```python
from build123d import *

# Parameters (mm, degrees)
SKETCH1_R           = 19
BOSS_EXTRUDE1_DEPTH = 32.5
CUT_EXTRUDE3_REACH  = 63.5
SKETCH2_R           = 5
CUT_EXTRUDE4_DEPTH  = 4.5


with BuildPart() as part:
    # Sketch1 → Boss-Extrude1 (new body, symmetric)
    with BuildSketch(Plane.XY):
        with BuildLine():
            Line((37.5, 28.5), (0, 28.5))
            ThreePointArc((0, 28.5), (-20.152543264, -20.152543264), (28.5, 0))
            Line((28.5, 0), (28.5, 7))
            ThreePointArc((28.5, 7), (31.428932188, 14.071067812), (38.5, 17))
            Line((38.5, 17), (97.5, 17))
            Line((97.5, 17), (97.5, 33))
            Line((97.5, 33), (37.5, 33))
            Line((37.5, 33), (37.5, 28.5))
        make_face()
        Circle(SKETCH1_R, mode=Mode.SUBTRACT)
    extrude(amount=BOSS_EXTRUDE1_DEPTH, both=True)

    # Sketch2 → Cut-Extrude3 (cut, up to next)
    with BuildSketch(Plane(origin=(0, 33, 0), x_dir=(1, 0, 0), z_dir=(0, 1, 0)), mode=Mode.PRIVATE) as cut_extrude3_sk1:
        with BuildLine():
            Line((97.5, 32.5), (50, 32.5))
            ThreePointArc((50, 32.5), (53.208349189, 32.08124561), (56.201736729, 30.853039277))
            Line((56.201736729, 30.853039277), (91.201736729, 10.853039277))
            ThreePointArc((91.201736729, 10.853039277), (95.811376122, 6.2740853), (97.5, 1.68e-07))
            Line((97.5, 1.68e-07), (97.5, 32.5))
        make_face()
    cut_extrude3_tool1 = extrude(cut_extrude3_sk1.sketch, amount=-CUT_EXTRUDE3_REACH, mode=Mode.PRIVATE) & part.part
    add(cut_extrude3_tool1.solids().sort_by_distance((82.925685, 33, -23.833798))[0], mode=Mode.SUBTRACT)
    # Sketch2 → Cut-Extrude3 (cut, up to next)
    with BuildSketch(Plane(origin=(0, 33, 0), x_dir=(1, 0, 0), z_dir=(0, 1, 0)), mode=Mode.PRIVATE) as cut_extrude3_sk2:
        with BuildLine():
            ThreePointArc((56.201736729, -30.853039277), (53.208349189, -32.08124561), (50, -32.5))
            Line((50, -32.5), (97.5, -32.5))
            Line((97.5, -32.5), (97.5, 1.68e-07))
            ThreePointArc((97.5, 1.68e-07), (95.811376206, -6.274085155), (91.201736729, -10.853039277))
            Line((91.201736729, -10.853039277), (56.201736729, -30.853039277))
        make_face()
    cut_extrude3_tool2 = extrude(cut_extrude3_sk2.sketch, amount=-CUT_EXTRUDE3_REACH, mode=Mode.PRIVATE) & part.part
    add(cut_extrude3_tool2.solids().sort_by_distance((82.925685, 33, 23.833798))[0], mode=Mode.SUBTRACT)
    # Sketch2 → Cut-Extrude3 (cut, up to next)
    with BuildSketch(Plane(origin=(0, 33, 0), x_dir=(1, 0, 0), z_dir=(0, 1, 0)), mode=Mode.PRIVATE) as cut_extrude3_sk3:
        with Locations((85, 0)):
            Circle(SKETCH2_R)
    cut_extrude3_tool3 = extrude(cut_extrude3_sk3.sketch, amount=-CUT_EXTRUDE3_REACH, mode=Mode.PRIVATE) & part.part
    add(cut_extrude3_tool3.solids().sort_by_distance((85, 33, 0))[0], mode=Mode.SUBTRACT)
    # Sketch2 → Cut-Extrude3 (cut, up to next)
    with BuildSketch(Plane(origin=(0, 33, 0), x_dir=(1, 0, 0), z_dir=(0, 1, 0)), mode=Mode.PRIVATE) as cut_extrude3_sk4:
        with Locations((50, 20)):
            Circle(SKETCH2_R)
    cut_extrude3_tool4 = extrude(cut_extrude3_sk4.sketch, amount=-CUT_EXTRUDE3_REACH, mode=Mode.PRIVATE) & part.part
    add(cut_extrude3_tool4.solids().sort_by_distance((50, 33, -20))[0], mode=Mode.SUBTRACT)
    # Sketch2 → Cut-Extrude3 (cut, up to next)
    with BuildSketch(Plane(origin=(0, 33, 0), x_dir=(1, 0, 0), z_dir=(0, 1, 0)), mode=Mode.PRIVATE) as cut_extrude3_sk5:
        with Locations((50, -20)):
            Circle(SKETCH2_R)
    cut_extrude3_tool5 = extrude(cut_extrude3_sk5.sketch, amount=-CUT_EXTRUDE3_REACH, mode=Mode.PRIVATE) & part.part
    add(cut_extrude3_tool5.solids().sort_by_distance((50, 33, 20))[0], mode=Mode.SUBTRACT)

    # Sketch2_4 → Cut-Extrude4 (cut)
    with BuildSketch(Plane(origin=(0, 33, 0), x_dir=(1, 0, 0), z_dir=(0, 1, 0))):
        with BuildLine():
            ThreePointArc((50, -32.5), (41.161165235, -28.838834765), (37.5, -20))
            Line((37.5, -20), (37.5, -32.5))
            Line((37.5, -32.5), (50, -32.5))
        make_face()
        with BuildLine():
            Line((37.5, 32.5), (37.5, 20))
            ThreePointArc((37.5, 20), (41.161165235, 28.838834765), (50, 32.5))
            Line((50, 32.5), (37.5, 32.5))
        make_face()
    extrude(amount=-CUT_EXTRUDE4_DEPTH, mode=Mode.SUBTRACT)


solid = part.part
```
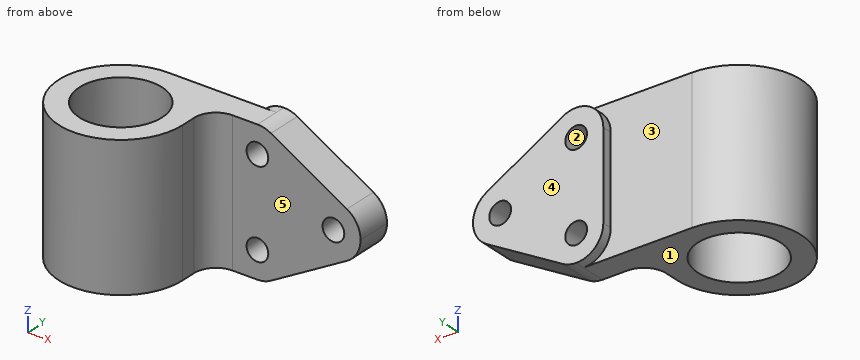
Design review of the part built by this model. Coordinates are the model's own, in mm. Face numbers are marked on the shaded views. A direction names the side the tool comes from. Give positions to 0.01 mm unless a question says otherwise; leave off trailing zeros. Order: outer loops, then holes, each group sorted by start corner. A loop starts at its lowest first (then second) coordinate and runs counter-clockwise, first axis right, second up. Notation, with made-up numbers: (89.25, 62) -> (116.25, 62) arc R33 ccw to (116.25, 92) -> close; hole circle Ø2 at (38.5, 52). An arc over 180 degrees is marked (long way). Write each question's results on one line, items separated by ' | '. Start each with the question number.
Q1. Add section B-B on z = -7.5. Give the boundary of the cut face in (x, y).
Q2. Add section A-A on z = 18.5. Give the boundary of the cut face in (x, y).
Q3. Add section C-C on y = -5.5. Give the boundary of the cut face in (x, z).
Q4. Machinability: for the marked faces 4 and 5, which of the approach directions +Z, -Z, +X, -X, +Y, -Y give a long, thin tool a straight path to every point of the face, cutting with its end or side? Answer none if there is none.
Q5. Wall thickness on L1, parallel to Z at x = 50, y = 24; L2, parallel to X at y = 1, z = 19.5; L3, parallel to Y at x = 53, z = 0: over which ranges is each line inside the solid? List them lowest first. Write a range as from..to.
Q6. Add section D-D on x = 11. Give the boundary of the cut face in (y, z).
Q7. Mouldability with a two-part tool opening along Z and no side actions: class the marked faces 1, 2 and 3 as +Z half, -Z half, draft (parallel to the pull), parting line (faces both ways), or undercut.
Q8. For pin 1 (1.5 mm diameter, centred on x = 9.5, z = 3, fed in from -Y); pin 2 (3.5 mm diameter, centred on y = 3.5, z = 2, fed in from +X); pin 3 (16 mm diameter, centred on x = 50, z = 20, fed in from -Y), all flat-tipped, find the tip position at first contact; note any pin that passes through.
Found:
1) outline: (0, 28.5) arc R28.5 ccw (long way) to (28.5, 0) -> (28.5, 7) arc R10 cw to (38.5, 17) -> (95, 17) -> (95, 33) -> (37.5, 33) -> (37.5, 28.5) -> close; hole circle Ø38 at (0, 0)
2) outline: (0, 28.5) arc R28.5 ccw (long way) to (28.5, 0) -> (28.5, 7) arc R10 cw to (38.5, 17) -> (45.23, 17) -> (45.23, 33) -> (37.5, 33) -> (37.5, 28.5) -> close; (54.77, 17) -> (77.82, 17) -> (77.82, 33) -> (54.77, 33) -> close; hole circle Ø38 at (0, 0)
3) outline: (-27.96, -32.5) -> (-18.19, -32.5) -> (-18.19, 32.5) -> (-27.96, 32.5) -> close; (18.19, -32.5) -> (27.96, -32.5) -> (27.96, 32.5) -> (18.19, 32.5) -> close
4) face 4: +Z, -Z, +X, -X, +Y | face 5: +Z, -Z, +X, -Y
5) L1: z = -32.5..-25, -15..15, 25..32.5 | L2: x = -28.48..-18.97, 18.97..28.5 | L3: y = 17..33
6) outline: (-26.29, -32.5) -> (-15.49, -32.5) -> (-15.49, 32.5) -> (-26.29, 32.5) -> close; (15.49, -32.5) -> (28.5, -32.5) -> (28.5, 32.5) -> (15.49, 32.5) -> close
7) face 1: -Z half | face 2: undercut | face 3: draft
8) pin 1: stops at y = -27.12 | pin 2: stops at x = 28.5 | pin 3: stops at y = 17
